Here's the drawing with two shaded views (mm, measured from the low corner). I have some questions. A direction names the side the tool comes from. Coordinates: 2 decimals unless noted, no trailing zeros. Loops run counter-clockwise (first coordinate to the right, second up) from the corner with the lowest first, then second, coordinate; pieces in that order, holes last. Notation, with made-up numbers: (35, 5.25) -> (80, 5.25) arc R7 ccw to (80, 11.25) -> close; hole circle Ø3 at (-35, -21.75). An arc over 180 degrees is marked (long way). Answer as a JSON object with one key per item and string values. Group by question number.
Q1. I need wall thicknesses on line 1 (X direction, y = 9, z = 25) (1 decimal); line 2 (Z direction, x = 139, y = 14); line 3 (Z direction, x = 102.5, y = 4.25). Which ranges of each line are inside material? Lowest first, please.
Q2. I want a section at B-B on y = 22.25. Write out the boundary of the cut face in (x, z) (1 decimal).
Q3. I want a section at A-A on z = 46. Write out the boundary of the cut face in (x, y) (1 decimal).
Q4. I'm going to push flat-ended pins straight in: pin 1 (8 mm diameter, centred on x = 125, z = 64.5, fed in from -Y); pin 2 (6 mm diameter, centred on x = 67.5, y = 9.5, fed in from +Z). Where does each tip first touch, or does it pass through?
Q5. I want a section at C-C on x = 38. Write out the boundary of the cut face in (y, z).
Q6. I want a section at D-D on x = 135.5. Write out the boundary of the cut face in (y, z), then the cut area to 3 significant figures.
Q7. Thinking about a two-plate mould opening in X: for the marked faces 3, 4 and 5, which applies, released by +X, released by -X, zero draft, split by the parting line, or undercut?
Q8. On a 3-axis mill with a long thin cutter (end or side, diameter ignored), from which of +Z, -Z, +X, -X, +Y, -Y can I reach the whole of each face in a straight line? I mean the marked faces 1 and 2. Say none if no direction works.
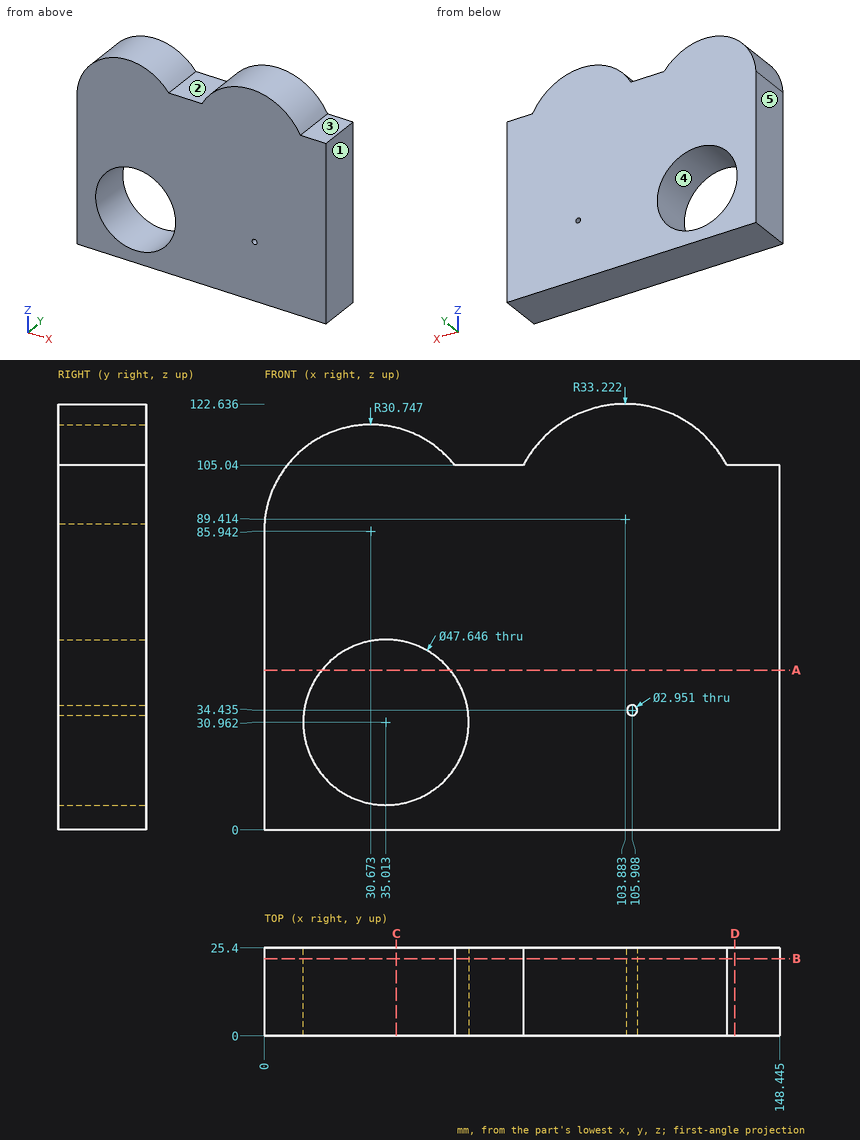
Result set:
{
 "1": {"line 1": "x = 0 to 11.9, 58.1 to 148.4", "line 2": "z = 0 to 105.04", "line 3": "z = 0 to 122.61"},
 "2": {"outline": "(0, 0) -> (148.4, 0) -> (148.4, 105) -> (133.2, 105) arc R33.2 ccw to (74.6, 105) -> (54.8, 105) arc R30.7 ccw to (0, 88.1) -> close; hole circle Ø47.6 at (35, 31); hole circle Ø3 at (105.9, 34.4)"},
 "3": {"outline": "(0, 0) -> (16.5, 0) -> (16.5, 25.4) -> (0, 25.4) -> close; (53.5, 0) -> (148.4, 0) -> (148.4, 25.4) -> (53.5, 25.4) -> close"},
 "4": {"pin 1": "stops at y = 0", "pin 2": "stops at z = 105.04"},
 "5": {"outline": "(0, 0) -> (25.4, 0) -> (25.4, 7.33) -> (0, 7.33) -> close; (0, 54.6) -> (25.4, 54.6) -> (25.4, 115.8) -> (0, 115.8) -> close"},
 "6": {"outline": "(0, 0) -> (25.4, 0) -> (25.4, 105.04) -> (0, 105.04) -> close", "area": "2,670 mm²"},
 "7": {"face 3": "zero draft", "face 4": "undercut", "face 5": "released by -X"},
 "8": {"face 1": "+Z, -Z, +X, +Y, -Y", "face 2": "+Z, +Y, -Y"}
}
